Source: three-view drawing plus pictorial views. Frame: mm from the lowest corner of the part. Give positions to 0.01 mm unless a question says otherwise; leave off trailing zeros. Loops run counter-clockwise (first coordinate to the right, second up) from the corner with the lowest first, then second, coordinate; pieces in that order, holes last. Notation, with made-up numbers: (31.5, -21) - (40.5, -21) arc R19 ccw to (40.5, 4) - close; hole circle Ø2 at (86.25, 62.25). An arc over 180 degrees is marked (long way). One line per item, written item: value.
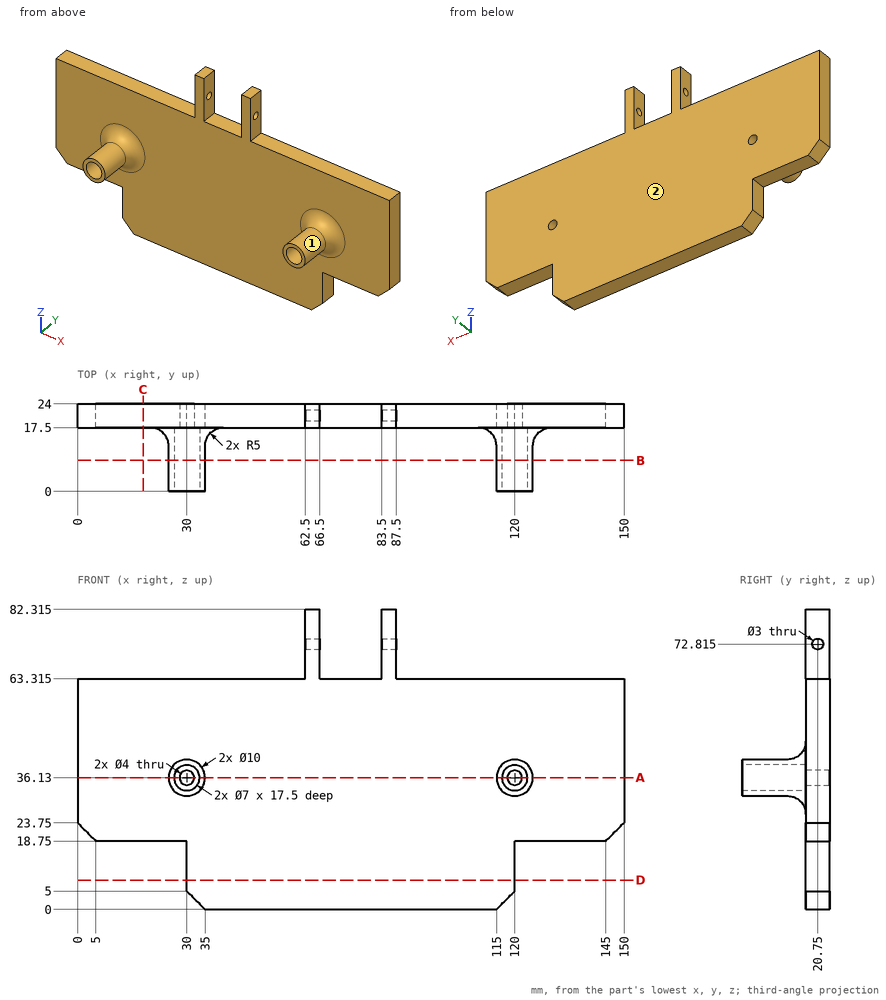
Item 1: Draft query along X for the marked faces 1 and 2. Return one class per face: pulls with the +X half, pulls with the -X half, needs draft (parallel to the pull), parting line crosses it, or undercut.
Verdict:
face 1: undercut
face 2: needs draft
Item 2: Section B-B, the plane y = 8.5. Output: boundary loops of the cut face in (x, z), and give its area (3 significant figures).
Verdict:
outline: circle Ø10 at (30, 36.13); circle Ø10 at (120, 36.13); hole circle Ø7 at (30, 36.13); hole circle Ø7 at (120, 36.13)
area: 80.1 mm^2
Item 3: Section D-D, the plane z = 8. Output: boundary loops of the cut face in (x, y).
Verdict:
outline: (30, 17.5) - (120, 17.5) - (120, 24) - (30, 24) - close
Item 4: Section C-C, the plane x = 18. Output: boundary loops of the cut face in (y, z) (3 decimals).
Verdict:
outline: (17.5, 18.75) - (24, 18.75) - (24, 63.315) - (17.5, 63.315) - close
Item 5: Pin query (flat end, axial travel): P1, Ø7, axis at x = 112.5, y = 21.5, coming from the +Z side (3 decimals); P2, Ø2, axis at y = 21.5, z = 71.5, coming from the +X side; P3, Ø3, axis at y = 20, z = 33.5, coming from the -X side; P4, Ø4, axis at x = 116.5, y = 13, coming from the +Z side. Return the tip coordinate at first contact, or that it passes through.
Verdict:
P1: stops at z = 63.315
P2: stops at x = 87.5
P3: stops at x = 0
P4: stops at z = 41.09
Item 6: Section A-A, the plane z = 36.13. Count the separate pieces of the cut face and the enclosed holes in it, and give its area (3 significant figures).
Verdict:
separate pieces: 3
enclosed holes: 0
area: 1,050 mm^2
Item 7: Material intervals for L1, parallel to X at y = 9.25, z = 36.13; L2, parallel to X at y = 18.25, z = 12; L3, parallel to Z at x = 73.5, y = 21 (3 decimals), sorted ascending.
Verdict:
L1: x = 25 to 26.5, 33.5 to 35, 115 to 116.5, 123.5 to 125
L2: x = 30 to 120
L3: z = 0 to 63.315
